Check sheet for the modelled part. Datum: model origin and axes. Units: mm. Face numbers are marked on the shaded views. A direction names the side the tool comes from. Coordinates: 2 decimals unless noted, no trailing zeros. Loops run counter-clockwise (first coordinate to the right, second up) from the corner with the lowest first, then second, coordinate; pieces in that order, holes last.
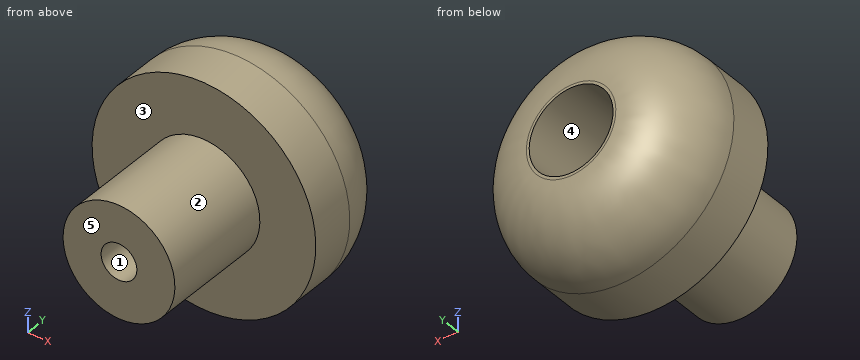
```python
from build123d import *

# Parameters (mm, degrees)
SZKIC1_R                    = 10
DODANIE_WYCI_GNI_CIE1_DEPTH = 10
ZAOKR_GLENIE1_R             = 6
SZKIC2_R                    = 5
DODANIE_WYCI_GNI_CIE2_DEPTH = 10
SZKIC3_R                    = 3.75
WYTNIJ_WYCI_GNI_CIE1_DEPTH  = 8
WYTNIJ_WYCI_GNI_CIE2_REACH  = 26.495
SZKIC4_R                    = 1.6


with BuildPart() as part:
    # Szkic1 → Dodanie-wyciągnięcie1 (new body)
    with BuildSketch(Plane(origin=(0, 0, 0), x_dir=(1, 0, 0), z_dir=(0, 1, 0))):
        with Locations(Location((0, 0, 0), (0, 0, 270))):
            Circle(SZKIC1_R)
    extrude(amount=DODANIE_WYCI_GNI_CIE1_DEPTH)

    # Zaokrąglenie1
    zaokr_glenie1_edges = [part.edges().sort_by_distance(p)[0] for p in [
        (0, 10, -10),
    ]]
    fillet(zaokr_glenie1_edges, radius=ZAOKR_GLENIE1_R)

    # Szkic2 → Dodanie-wyciągnięcie2 (add)
    with BuildSketch(Plane.XZ):
        with Locations(Location((0, 0, 0), (0, 0, 270))):
            Circle(SZKIC2_R)
    extrude(amount=DODANIE_WYCI_GNI_CIE2_DEPTH)

    # Szkic3 → Wytnij-wyciągnięcie1 (cut)
    with BuildSketch(Plane(origin=(0, 10, 0), x_dir=(1, 0, 0), z_dir=(0, 1, 0))):
        with Locations(Location((0, 0, 0), (0, 0, 270))):
            Circle(SZKIC3_R)
    extrude(amount=-WYTNIJ_WYCI_GNI_CIE1_DEPTH, mode=Mode.SUBTRACT)

    # Szkic4 → Wytnij-wyciągnięcie2 (cut, up to next)
    with BuildSketch(Plane.XZ.offset(10), mode=Mode.PRIVATE) as wytnij_wyci_gni_cie2_sk1:
        with Locations(Location((0, 0, 0), (0, 0, 270))):
            Circle(SZKIC4_R)
    wytnij_wyci_gni_cie2_tool1 = extrude(wytnij_wyci_gni_cie2_sk1.sketch, amount=-WYTNIJ_WYCI_GNI_CIE2_REACH, mode=Mode.PRIVATE) & part.part
    add(wytnij_wyci_gni_cie2_tool1.solids().sort_by_distance((0, -10, 0))[0], mode=Mode.SUBTRACT)


solid = part.part
```
1) Mould release check, pull along Z, two halves, no side actions. Record for the marked faces 1, 2 and 3: +Z half, -Z half, draft (parallel to the pull), parting line (faces both ways), or undercut.
Answer sheet:
face 1: undercut
face 2: parting line
face 3: draft
2) Section check A-A on y = -7. Enter the section's corners in (x, z).
Answer sheet:
outline: circle Ø10 at (0, 0); hole circle Ø3.2 at (0, 0)
3) Depth check by flat-ended pin: pin 1 (3.5 mm diameter, centred on x = 0, z = 0, fed in from +Y); pin 2 (1 mm diameter, centred on x = 4, z = 5, fed in from +Y); pin 3 (10 mm diameter, centred on x = -6, y = 2, fed in from -Z). Enter the tip coordinate at first touch or a pass-through.
Answer sheet:
pin 1: stops at y = 2
pin 2: stops at y = 9.69
pin 3: stops at z = -9.95
4) Scan lines: line 1 (X direction, y = -5.5, z = 0); line 2 (X direction, y = 9, z = 2.5); line 3 (Y direction, x = -0.75, z = -1.5). Record each from-to range of solid material in increasing order.
Answer sheet:
line 1: x = -5 to -1.6, 1.6 to 5
line 2: x = -6.88 to -2.8, 2.8 to 6.88
line 3: y = -10 to 2
5) Set-up check for the marked faces 4 and 5: record each of +Z, -Z, +X, -X, +Y, -Y from which the full face is reachable in a straight line by a thin tool's end or side.
Answer sheet:
face 4: +Y
face 5: +Z, -Z, +X, -X, -Y
